Source: CAD feature listing. Evaluate the final solid. Frame: model axes, mm. A direction names the side the tool comes from. Coordinates: 2 decimals unless noted, no trailing zeros. Loops run counter-clockwise (first coordinate to the right, second up) from the corner with the lowest first, then second, coordinate; pieces in that order, holes last.
Item 1: Pin query (flat end, axial travel): pin 1 Ø2.5 at (y, z) = (-9, 20.5) entering from -X; pin 2 Ø8 at (x, y) = (-12.5, -11.5) entering from -Z; pin 3 Ø2 at (x, y) = (21.5, -12.5) entering from +Z; pin 4 Ø2.5 at (x, y) = (17.399, -17.4) entering from -Z. Return the tip coordinate at first contact, or that it passes through.
Item 2: Reachability of faces 4 (the flat face through (23.812, -10, 16)), 5 (the flat face through (-16.5, -11, 93)), 6 (the flat face through (17, -12, 0)) from +Z, -Z, +X, -X, +Y, -Y: full face, straight path, thin tool, end or side. Return the list, or none.
Item 3: Pull-direction query (Y, two-part tool) for faces 1 (the cylindrical face through (-22.992, -15.875, 3.899)), 2 (the flat face through (19, -16, -2.845)), 3 (the flat face through (0, -5, 44.45)); classes: +Y half, -Y half, draft (parallel to the pull), parting line (faces both ways), or undercut.
Item 4: Line query: probe 1 along X at (y, z) = (-10, 75.5); probe 2 along Z at (x, y) = (17.5, -4.25) (3 decimals); probe 3 along Y at (x, z) = (0, 104) (3 decimals). Output: solid intervals per line, ascending.
Item 5: Section query B-B, the plane x = -3.5. Return the cut outline in (y, z) (3 decimals).
Item 6: Section query A-A, the plane z = 76. Return the cut outline in (x, y) (3 decimals).
```python
from build123d import *

# Parameters (mm, degrees)
SKETCH1_W                                     = 50.8
SKETCH1_H                                     = 25.4
BASE_FLANGE1_DEPTH                            = 6.35
SKETCH22_W                                    = 50.8
SKETCH22_H                                    = 160
BOSS_EXTRUDE1_DEPTH                           = 3.175
GUSSET1_START                                 = -22.225
GUSSET1_DEPTH                                 = 1.5875
CBORE_FOR_4_SOCKET_HEAD_CAP_SCREW1_AT_2_COUNT = 2
CBORE_FOR_4_SOCKET_HEAD_CAP_SCREW1_AT_2_PITCH = 34.798
SKETCH12_W                                    = 26
SKETCH12_H                                    = 28.575
CUT_EXTRUDE1_DEPTH                            = 50.8
SKETCH13_W                                    = 33.6375
SKETCH13_H                                    = 12.7
CUT_EXTRUDE2_DEPTH                            = 50.8
CBORE_FOR_2_SOCKET_HEAD_CAP_SCREW1_AT_2_COUNT = 2
CBORE_FOR_2_SOCKET_HEAD_CAP_SCREW1_AT_2_PITCH = 33.801054175
CBORE_FOR_2_SOCKET_HEAD_CAP_SCREW1_AT_3_COUNT = 2
CBORE_FOR_2_SOCKET_HEAD_CAP_SCREW1_AT_3_PITCH = 33.801054175
EXTRUDE_THIN1_DEPTH                           = 10
SKETCH25_W                                    = 3.175
SKETCH25_H                                    = 31.5
EXTRUDE_THIN2_DEPTH                           = 10
SKETCH17_OUTSIDE_W                            = 86.756
SKETCH17_OUTSIDE_H                            = 61.356
SKETCH17_OUTSIDE_R                            = 27.94
CUT_EXTRUDE3_DEPTH                            = 165.504378741
FILLET1_R                                     = 10
FILLET2_R                                     = 4
SKETCH24_W                                    = 31
SKETCH24_H                                    = 1.75
CUT_EXTRUDE4_DEPTH                            = 125.15


# Read off the part's stored shape, not the designer's step: Gusset1
# Sheet-metal steps are written as plain solids
with BuildPart() as part:
    # Sketch1 → Base-Flange1 (new body)
    with BuildSketch(Plane.XY):
        with Locations((0, -15.875)):
            Rectangle(SKETCH1_W, SKETCH1_H)
    extrude(amount=-BASE_FLANGE1_DEPTH)

    # Sketch22 → Boss-Extrude1 (add)
    with BuildSketch(Plane(origin=(0, -3.175, 0), x_dir=(1, 0, 0), z_dir=(0, 1, 0))):
        with Locations((0, -73.65)):
            Rectangle(SKETCH22_W, SKETCH22_H)
    extrude(amount=-BOSS_EXTRUDE1_DEPTH)

    # Sketch11 → CBORE for #4 Socket Head Cap Screw1 (revolve, cut)
    with BuildSketch(Plane(origin=(-17.399, -17.4, 0), x_dir=(0, -1, 0), z_dir=(1, 0, 0))):
        Polygon((0, 0), (0, 6.351), (1.4732, 6.351), (1.4732, 2.8448), (2.77876, 2.8448), (2.77876, 0), align=None)
    cbore_for_4_socket_head_cap_screw1 = revolve(axis=Axis((-17.399, -17.4, 6.35), (0, 0, -1)), mode=Mode.SUBTRACT)

    # CBORE for #4 Socket Head Cap Screw1 at 2: CBORE for #4 Socket Head Cap Screw1 ×2
    with Locations(*[(i * CBORE_FOR_4_SOCKET_HEAD_CAP_SCREW1_AT_2_PITCH, 0, 0) for i in range(1, CBORE_FOR_4_SOCKET_HEAD_CAP_SCREW1_AT_2_COUNT)]):
        add(cbore_for_4_socket_head_cap_screw1, mode=Mode.SUBTRACT)

    # Sketch12 → Cut-Extrude1 (cut)
    with BuildSketch(Plane(origin=(0, 0, -6.35), x_dir=(-1, 0, 0), z_dir=(0, 0, -1))):
        with Locations((0, -14.2875)):
            Rectangle(SKETCH12_W, SKETCH12_H)
    extrude(amount=-CUT_EXTRUDE1_DEPTH, mode=Mode.SUBTRACT)


with BuildPart() as body_2:
    # Gusset1 outline → Gusset1 (new body)
    with BuildSketch(Plane.YZ.offset(GUSSET1_START)):
        Polygon((-16.35, 5), (-16.35, 0), (-6.35, 0), (-6.35, 30), (-10.35, 30), align=None)
    gusset1 = extrude(amount=GUSSET1_DEPTH)


with BuildPart() as part_1:
    add(part.part)

    # Mirror2: Gusset1 across plane
    add(gusset1.mirror(Plane(origin=(0, 0, 0), x_dir=(0, 0, 1), z_dir=(1, 0, 0))))

    # Sketch13 → Cut-Extrude2 (cut)
    with BuildSketch(Plane.XZ.offset(6.35)):
        with Locations((3.81875, 15.335)):
            Rectangle(SKETCH13_W, SKETCH13_H)
    extrude(amount=-CUT_EXTRUDE2_DEPTH, mode=Mode.SUBTRACT)

    # Sketch16 → CBORE for #2 Socket Head Cap Screw1 (revolve, cut)
    with BuildSketch(Plane(origin=(-16.256, -3.175, 15.335), x_dir=(0, 0, 1), z_dir=(1, 0, 0))):
        Polygon((0, 0), (0, 17.242569267), (1.2192, 16.51), (1.2192, 2.1844), (2.38125, 2.1844), (2.38125, 0), align=None)
    cbore_for_2_socket_head_cap_screw1 = revolve(axis=Axis((-16.256, 3.175, 15.335), (0, -1, 0)), mode=Mode.SUBTRACT)

    # CBORE for #2 Socket Head Cap Screw1 at 2: CBORE for #2 Socket Head Cap Screw1 ×2
    with Locations(*[Vector(0.9618634919315714, 0, 0.27352993051804053) * (i * CBORE_FOR_2_SOCKET_HEAD_CAP_SCREW1_AT_2_PITCH) for i in range(1, CBORE_FOR_2_SOCKET_HEAD_CAP_SCREW1_AT_2_COUNT)]):
        add(cbore_for_2_socket_head_cap_screw1, mode=Mode.SUBTRACT)

    # CBORE for #2 Socket Head Cap Screw1 at 3: CBORE for #2 Socket Head Cap Screw1 ×2
    with Locations(*[Vector(0.9618634919315714, 0, -0.2735299305180405) * (i * CBORE_FOR_2_SOCKET_HEAD_CAP_SCREW1_AT_3_PITCH) for i in range(1, CBORE_FOR_2_SOCKET_HEAD_CAP_SCREW1_AT_3_COUNT)]):
        add(cbore_for_2_socket_head_cap_screw1, mode=Mode.SUBTRACT)

    add(body_2.part)  # Extrude-Thin1 merges body 2
    # Sketch23 → Extrude-Thin1 (add)
    with BuildSketch(Plane.XZ.offset(6.35)):
        Polygon((-22.225, 28.5), (-13.5, 28.5), (-13.5, 153.65), (-16.5, 153.65), (-16.5, 31.5), (-22.225, 31.5), align=None)
        Polygon((13.5, 153.65), (13.5, 28.5), (22.225, 28.5), (22.225, 31.5), (16.5, 31.5), (16.5, 153.65), align=None)
    extrude(amount=EXTRUDE_THIN1_DEPTH)

    # Sketch25 → Extrude-Thin2 (add)
    with BuildSketch(Plane.XZ.offset(6.35)):
        with Locations((-22.225, 15.75)):
            Rectangle(SKETCH25_W, SKETCH25_H)
        with Locations((22.225, 15.75)):
            Rectangle(SKETCH25_W, SKETCH25_H)
    extrude(amount=EXTRUDE_THIN2_DEPTH)

    # Sketch17 outside → Cut-Extrude3 (cut, through all)
    with BuildSketch(Plane(origin=(0, 0, -6.35), x_dir=(-1, 0, 0), z_dir=(0, 0, -1))):
        with Locations((0, -15.875)):
            Rectangle(SKETCH17_OUTSIDE_W, SKETCH17_OUTSIDE_H)
        Circle(SKETCH17_OUTSIDE_R, mode=Mode.SUBTRACT)
    extrude(amount=-CUT_EXTRUDE3_DEPTH, mode=Mode.SUBTRACT)

    # Fillet1
    fillet1_edges = [part_1.edges().sort_by_distance(p)[0] for p in [
        (-25.4, -11.639742265, -3.175),
        (25.4, -11.639742265, -3.175),
    ]]
    fillet(fillet1_edges, radius=FILLET1_R)

    # Fillet2
    fillet2_edges = [part_1.edges().sort_by_distance(p)[0] for p in [
        (-13, -24.731429397, -3.175),
        (13, -24.731429397, -3.175),
    ]]
    fillet(fillet2_edges, radius=FILLET2_R)

    # Sketch24 → Cut-Extrude4 (cut)
    with BuildSketch(Plane.XY.offset(153.65)):
        with Locations((0, -11.225)):
            Rectangle(SKETCH24_W, SKETCH24_H)
    extrude(amount=-CUT_EXTRUDE4_DEPTH, mode=Mode.SUBTRACT)


solid = part_1.part
```
Verdict:
1. pin 1: stops at x = -23.81
1. pin 2: stops at z = -6.35
1. pin 3: stops at z = 31.5
1. pin 4: stops at z = 28.5
2. face 4: +Z, +X, -Y
2. face 5: +Z, -X, -Y
2. face 6: -Y
3. face 1: -Y half
3. face 2: undercut
3. face 3: draft
4. probe 1: x = -16.5 to -13.5, 13.5 to 16.5
4. probe 2: z = -6.35 to 4.059, 8.12 to 8.985, 21.685 to 22.55, 26.611 to 153.65
4. probe 3: y = -6.35 to -3.175
5. outline: (-6.35, 44.45) - (-3.175, 44.45) - (-3.175, 153.65) - (-6.35, 153.65) - close
6. outline: (-25.4, -6.35) - (-16.5, -6.35) - (-16.5, -16.35) - (-13.5, -16.35) - (-13.5, -12.1) - (-15.5, -12.1) - (-15.5, -10.35) - (-13.5, -10.35) - (-13.5, -6.35) - (13.5, -6.35) - (13.5, -10.35) - (15.5, -10.35) - (15.5, -12.1) - (13.5, -12.1) - (13.5, -16.35) - (16.5, -16.35) - (16.5, -6.35) - (25.4, -6.35) - (25.4, -3.175) - (-25.4, -3.175) - close
